Build history of the part. All positions in model axes, mm. Give positions to 0.01 mm unless a question says otherwise; leave off trailing zeros. Write each loop counter-clockwise with the first axis right and the second up, starting at its lowest first coordinate (ties: lowest second). Pieces come first, ordered by that corner, then holes. Notation, with made-up numbers: M 83.5,8 L 140.5,8 A30 ccw 140.5,45 Z; hole C 10,23.25 d9. An arc over 180 degrees is marked long. Return JSON: item names as keys, results as strings. Group by question number.
Q1. Band-saw the part on A-A, the plane z = -20. Give the cut face in (x, y).
Q2. Wall check: probe 1 along Y at (x, z) = (35.5, 5); probe 2 along X at (y, z) = (37.5, -5); probe 3 along Y at (x, z) = (35.5, 2.5). Give the ranges that are in metal, low to high.
Q3. Band-saw the part on C-C, the plane x = -38. Give the cut face in (y, z).
Q4. Flat gauge pins, fed straight in: pin 1 Ø12 at (x, z) = (13, -16) entering from +Y; pin 2 Ø3 at (x, z) = (43.5, -17) entering from +Y; pin 3 Ø8 at (x, y) = (24, -36.5) entering from +Z. Where does each tip first touch, or does it go through?
Q5. Band-saw the part on B-B, the plane y = -18.5. Give the cut face in (x, z).
Q6. Band-saw the part on D-D, the plane z = 46. Give the cut face in (x, y), then the cut area to 3 significant figures.
from build123d import *


with BuildPart() as f1:
    # F0 (on Front) → F1 (revolve)
    with BuildSketch(Plane.XZ):
        with BuildLine():
            Line((0, 38.1), (0, -38.1))
            ThreePointArc((0, -38.1), (38.1, 0), (0, 38.1))
        make_face()
    revolve(axis=Axis((0, 0, 0), (0, 0, -1)))

    # F2 (on Right) → F3 (revolve)
    with BuildSketch(Plane.YZ):
        with BuildLine():
            Line((0, 63.135213), (0, 12.335213))
            ThreePointArc((0, 12.335213), (25.4, 37.735213), (0, 63.135213))
        make_face()
    revolve(axis=Axis((0, 0, 37.735213), (0, 0, -1)))

    # F2 (on Right) → F4 (revolve)
    with BuildSketch(Plane.YZ):
        with BuildLine():
            ThreePointArc((-12.335213, 0), (-37.735213, 25.4), (-63.135213, 0))
            Line((-63.135213, 0), (-12.335213, 0))
        make_face()
    revolve(axis=Axis((0, -37.735213, 0), (0, 1, 0)))

    # F2 (on Right) → F5 (revolve)
    with BuildSketch(Plane.YZ):
        with BuildLine():
            ThreePointArc((0, -12.335213), (-25.4, -37.735213), (0, -63.135213))
            Line((0, -63.135213), (0, -12.335213))
        make_face()
    revolve(axis=Axis((0, 0, -37.735213), (0, 0, 1)))

    # F2 (on Right) → F6 (revolve)
    with BuildSketch(Plane.YZ):
        with BuildLine():
            ThreePointArc((12.335213, 0), (37.735213, -25.4), (63.135213, 0))
            Line((63.135213, 0), (12.335213, 0))
        make_face()
    revolve(axis=Axis((0, 37.735213, 0), (0, -1, 0)))

    # F7 (on Front) → F8 (revolve)
    with BuildSketch(Plane.XZ):
        with BuildLine():
            Line((-63.412182, 0), (-12.612182, 0))
            ThreePointArc((-12.612182, 0), (-38.012182, 25.4), (-63.412182, 0))
        make_face()
    revolve(axis=Axis((-38.012182, 0, 0), (1, 0, 0)))

    # F7 (on Front) → F9 (revolve)
    with BuildSketch(Plane.XZ):
        with BuildLine():
            Line((12.612182, 0), (63.412182, 0))
            ThreePointArc((63.412182, 0), (38.012182, 25.4), (12.612182, 0))
        make_face()
    revolve(axis=Axis((38.012182, 0, 0), (-1, 0, 0)))


solid = f1.part
From the geometry:
{
 "1": {"outline": "M -29.61,-13.21 A32.43 ccw -13.35,-29.55 A15.66 ccw long 13.35,-29.55 A32.43 ccw 29.61,-13.21 A15.66 ccw long 29.61,13.21 A32.43 ccw 13.35,29.55 A15.66 ccw long -13.35,29.55 A32.43 ccw -29.61,13.21 A15.66 ccw long Z"},
 "2": {"probe 1": "y = -24.78 to 24.78", "probe 2": "x = -24.9 to 24.9", "probe 3": "y = -25.15 to 25.15"},
 "3": {"outline": "C 0,0 d50.8"},
 "4": {"pin 1": "stops at y = 58.51", "pin 2": "stops at y = 19.43", "pin 3": "stops at z = 15.62"},
 "5": {"outline": "M -29.61,-15.24 A33.31 ccw -15.36,-29.55 A17.4 ccw long 15.36,-29.55 A33.31 ccw 29.61,-15.24 A17.4 ccw long 29.61,15.24 A33.31 ccw 15.36,29.55 A17.4 ccw long -15.36,29.55 A33.31 ccw -29.61,15.24 A17.4 ccw long Z"},
 "6": {"outline": "C 0,0 d48.04", "area": "1,810 mm^2"}
}
